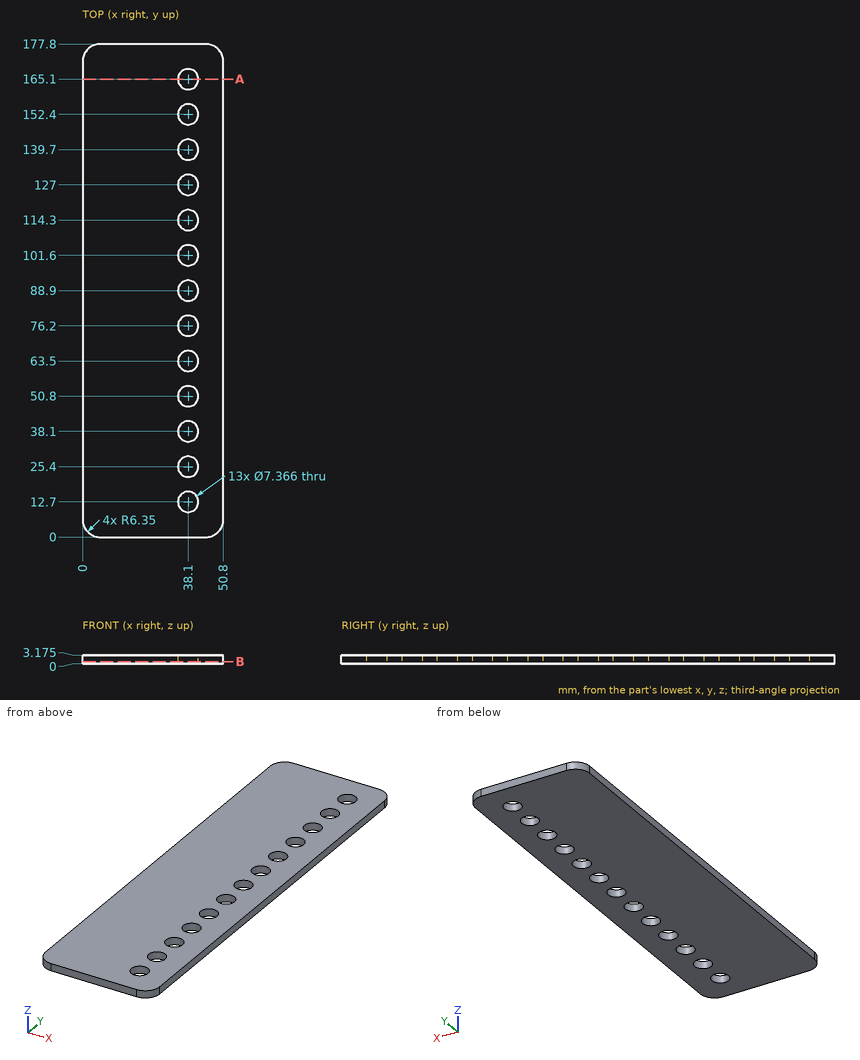
The drawing under review shows one solid part. Ordinate dimensions are in mm from its lowest x, y, z. Round coordinates to 2 decimals unless told otherwise and drop trailing zeros. Write each loop counter-clockwise with the first axis right and the second up, starting at its lowest first coordinate (ties: lowest second). Pieces come first, ordered by that corner, then holes. Notation, with made-up numbers: (-35, 63.5) - (-16, 63.5) arc R13 ccw to (-16, 78.5) - close; hole circle Ø11 at (37.25, 18). An arc over 180 degrees is marked (long way). Use a Markdown table: item, result. Add a question column.
1. Clearance check with a flat-ended pin moving along its axis: pin 1 (9.5 mm diameter, centred on x = 38.1, y = 127, fed in from +Z) (3 decimals). State where the tip first meets the part, or that it passes through.
2. We need section B-B (z = 0.85). Count the separate pieces of the cut face and the enclosed holes in it, then the cut area to 3 significant figures.
3. Wall thickness on probe 1 along X at (y, z) = (10.5, 1.65); probe 2 along X at (y, z) = (65.5, 2.9): over which ranges is each line inside the solid? List them lowest first.
4. We need section A-A (y = 165.1). State the section outline as (x, z) points (3 decimals).
Output:
| question | item | result |
|---|---|---|
| 1 | pin 1 | stops at z = 3.175 |
| 2 | separate pieces | 1 |
| 2 | enclosed holes | 13 |
| 2 | area | 8,440 mm2 |
| 3 | probe 1 | x = 0 to 35.15, 41.05 to 50.8 |
| 3 | probe 2 | x = 0 to 35.01, 41.19 to 50.8 |
| 4 | outline | (0, 0) - (34.417, 0) - (34.417, 3.175) - (0, 3.175) - close; (41.783, 0) - (50.8, 0) - (50.8, 3.175) - (41.783, 3.175) - close |
